The listing builds one solid part. Answer for the finished solid, in the listing's coordinates (mm). Face numbers are marked on the shaded views. A direction names the side the tool comes from. Give positions to 0.01 mm unless a question says otherwise; leave off trailing zeros. Loops run counter-clockwise (first coordinate to the right, second up) from the corner with the lowest first, then second, coordinate; pieces in that order, holes last. Notation, with made-up numbers: M -10.5,62.5 L -5.5,62.5 A18 cw -5.5,68.5 Z; hole C 63,45.5 d10. An arc over 180 degrees is marked long. One line per item, written item: value. Start each with the question number.
Q1. Consider L1, parallel to Y at x = 0, z = 30.65; L2, parallel to Y at x = 1, z = 68.5; L3, parallel to X at y = 16, z = 63.5. Determine where each line is inside the solid, lowest interval first.
Q2. Flat-ended cylindrical pins translate along their axes: pin 1 (11.5 mm diameter, centred on x = 0, y = 0, fed in from +Z); pin 2 (6 mm diameter, centred on x = 19.5, z = 30, fed in from +Y); pin 3 (5 mm diameter, centred on x = 4.5, z = 8, fed in from +Y). Find the tip coordinate at first contact, or state that the pin passes through.
Q3. The mould has two halves that part along Y. Classify the marked faces 3, 4 and 5: +Y half, -Y half, draft (parallel to the pull), parting line (faces both ways), or undercut.
Q4. A cutting plane is placed at D-D, the plane z = 33.5. Determine the outline of the cut face in (x, y), and give its area (3 significant figures).
Q5. A cutting plane is placed at C-C, the plane z = 54.5. Determine the outline of the cut face in (x, y), and give its area (3 significant figures).
Q6. For the marked faces 1 and 2, determine the directions among +Z, -Z, +X, -X, +Y, -Y from which every point of the face is accessible in a straight line to the end or side of a thin tool.
from build123d import *

# Parameters (mm, degrees)
F0_R     = 25
F0_R_2   = 5
F1_DEPTH = 45
F2_SIZE2 = 17
F2_SIZE  = 12.5
F3_R     = 25
F3_R_2   = 23
F4_DEPTH = 17
F5_R     = 28
F5_R_2   = 25
F5_R_3   = 24
F6_DEPTH = 10
F7_SIZE  = 2.99999
F8_SIZE2 = 30
F8_SIZE  = 5


# Not quite as in the source:
# - a fillet or chamfer is up to 0.001 mm smaller than in the source, because OpenCascade refuses the exact size


with BuildPart() as f1:
    # F0 (on Top) → F1 (new body)
    with BuildSketch(Plane.XY):
        Circle(F0_R)
        Circle(F0_R_2, mode=Mode.SUBTRACT)
    extrude(amount=F1_DEPTH)

    # F2
    f2_edges = [f1.edges().sort_by_distance(p)[0] for p in [
        (-5, 0, 45),
    ]]
    f2_side = f1.faces().sort_by_distance((-5, 0, 22.5))[0]
    chamfer(f2_edges, length=F2_SIZE, length2=F2_SIZE2, reference=f2_side)

    # F3 (on face) → F4 (join)
    with BuildSketch(Plane.XY.offset(45)):
        Circle(F3_R)
        Circle(F3_R_2, mode=Mode.SUBTRACT)
    extrude(amount=F4_DEPTH)

    # F5 (on face) → F6 (join)
    with BuildSketch(Plane.XY.offset(62)):
        Circle(F5_R)
        Circle(F5_R_2, mode=Mode.SUBTRACT)
        Circle(F5_R_2)
        Circle(F5_R_3, mode=Mode.SUBTRACT)
    extrude(amount=F6_DEPTH)

    # F7 (size 3 in the source; OpenCascade refuses exactly that, so slightly less here)
    f7_edges = [f1.edges().sort_by_distance(p)[0] for p in [
        (-25, 0, 62),
    ]]
    chamfer(f7_edges, length=F7_SIZE)

    # F8
    f8_edges = [f1.edges().sort_by_distance(p)[0] for p in [
        (-5, 0, 0),
    ]]
    f8_side = f1.faces().sort_by_distance((-24.292893, 0, 0))[0]
    chamfer(f8_edges, length=F8_SIZE, length2=F8_SIZE2, reference=f8_side)


solid = f1.part
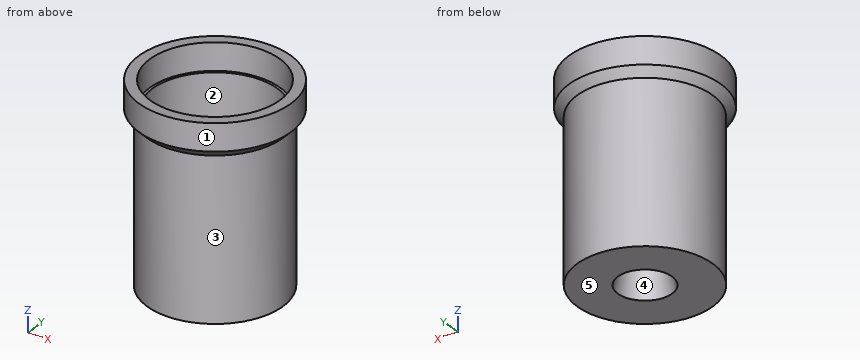
Answer block:
1. L1: -25 to -5, 5 to 25
1. L2: -27.98 to -23.98, 23.98 to 27.98
1. L3: -22.98 to -17.89, 17.89 to 22.98
2. pin 1: z = 33.05
2. pin 2: y = 18.78
2. pin 3: y = 24.92
3. face 3: parting line
3. face 4: undercut
3. face 5: draft
4. outline: C 0,0 d50; hole C 0,0 d12.72
4. area: 1,840 mm^2
5. outline: C 0,0 d50; hole C 0,0 d46
5. area: 302 mm^2
6. face 1: +Z, -Z
6. face 2: +Z
